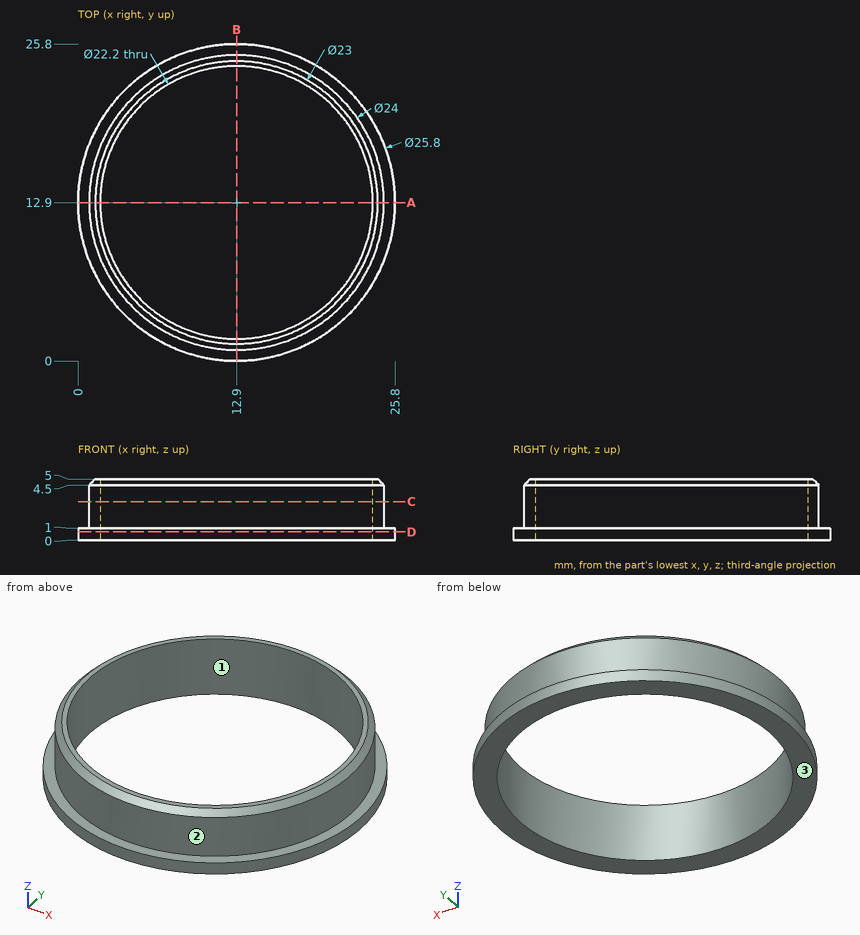
Source: three-view drawing plus pictorial views. Frame: mm from the lowest corner of the part. Coordinates: 2 decimals unless noted, no trailing zeros. Write each loop counter-clockwise with the first axis right and the second up, starting at its lowest first coordinate (ties: lowest second). Pieces come first, ordered by that corner, then holes. Notation, with made-up numbers: (-33.75, 46.25) - (-20.75, 46.25) arc R10 ccw to (-20.75, 61.25) - close; hole circle Ø6 at (-4, 54). An arc over 180 degrees is marked (long way). Return JSON: item names as keys, results as strings.
Item 1: Section query D-D (z = 0.7). Output: boundary loops of the cut face in (x, y).
Completed:
{"outline": "circle Ø25.8 at (12.9, 12.9); hole circle Ø22.2 at (12.9, 12.9)"}
Item 2: Pull-direction query (X, two-part tool) for the marked faces 1, 2 and 3; classes: +X half, -X half, draft (parallel to the pull), parting line (faces both ways), or undercut.
Completed:
{"face 1": "undercut", "face 2": "parting line", "face 3": "draft"}
Item 3: Pin query (flat end, axial travel): pin 1 Ø1 at (x, z) = (11, 4.5) entering from +Y; pin 2 Ø1 at (y, z) = (11, 3) entering from +X. Return the tip coordinate at first contact, or that it passes through.
Completed:
{"pin 1": "stops at y = 24.82", "pin 2": "stops at x = 24.82"}
Item 4: Line query: L1, parallel to Y at x = 12.9, z = 2.2; L2, parallel to X at y = 13, z = 0.2; L3, parallel to Z at x = 15, y = 24.75. Output: solid intervals per line, ascending.
Completed:
{"L1": "y = 0.9 to 1.8, 24 to 24.9", "L2": "x = 0 to 1.8, 24 to 25.8", "L3": "z = 0 to 1"}
Item 5: Section query C-C (z = 3.15). Output: boundary loops of the cut face in (x, y).
Completed:
{"outline": "circle Ø24 at (12.9, 12.9); hole circle Ø22.2 at (12.9, 12.9)"}
Item 6: Section query A-A (y = 12.9). Output: boundary loops of the cut face in (x, z), and give its area (4 significant figures).
Completed:
{"outline": "(0, 0) - (1.8, 0) - (1.8, 5) - (1.4, 5) - (0.9, 4.5) - (0.9, 1) - (0, 1) - close; (24, 0) - (25.8, 0) - (25.8, 1) - (24.9, 1) - (24.9, 4.5) - (24.4, 5) - (24, 5) - close", "area": "10.55 mm2"}
